Here's the drawing with two shaded views (mm, measured from the low corner). I have some questions. A direction names the side the tool comes from. Coordinates: 2 decimals unless noted, no trailing zeros. Write each loop counter-clockwise with the first axis right and the second up, starting at its lowest first coordinate (ties: lowest second). Pieces come first, ordered by that corner, then holes. Notation, with made-up numbers: (12, 70.5) -> (52, 70.5) arc R14 cw to (52, 92.5) -> close; hole circle Ø4 at (-32, 12.5). An arc over 180 degrees is marked (long way). Put each result on its own line as item: value.
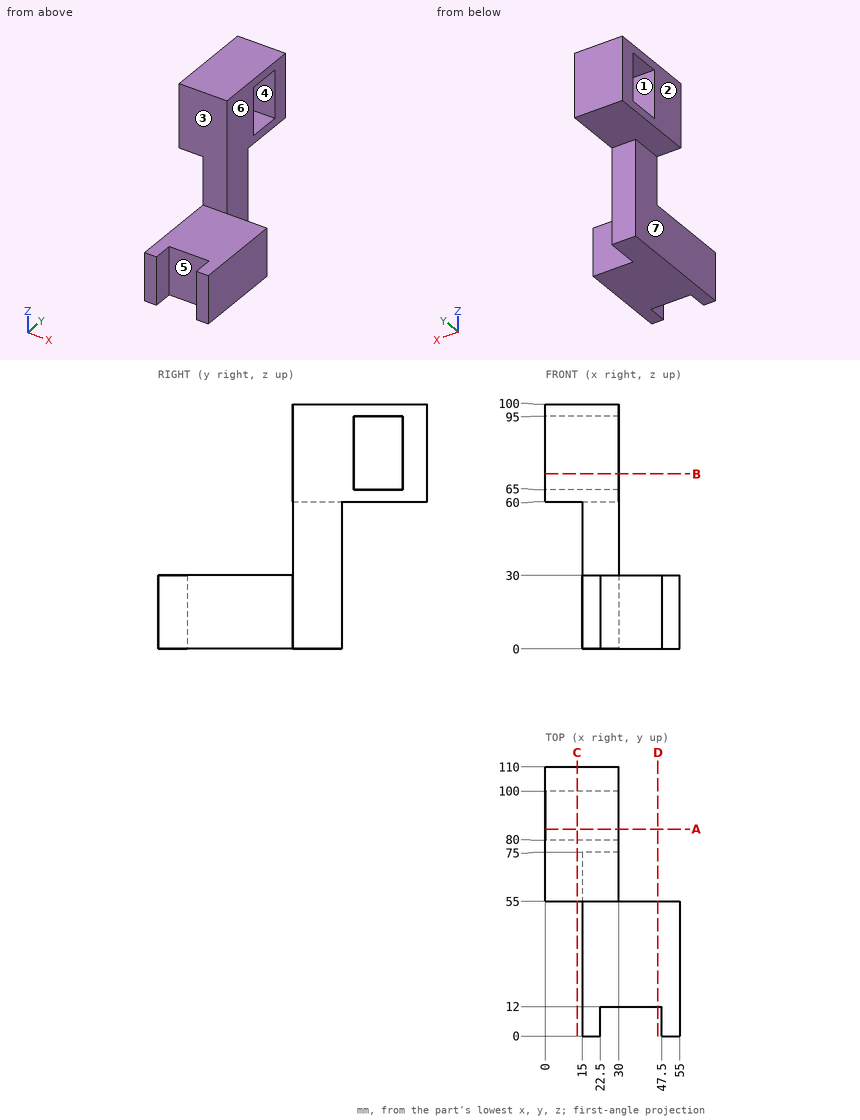
Item 1: For P1, Ø6, axis at y = 58.5, z = 26.5, coming from the +X side; P2, Ø16, axis at x = 9.5, y = 95, coming from the -Z side; P3, Ø15, axis at x = 10.5, z = 51, coming from the -Y side; P4, Ø12, axis at x = 24, z = 32.5, coming from the -Y side, each with a flat end and sliding along its axis, tell me the tip position at first contact or that it passes through.
Output:
P1: stops at x = 30
P2: stops at z = 60
P3: stops at y = 55
P4: stops at y = 0
Item 2: Please list where these lines run through material, in increasing order: line 1 along Y through (x, z) = (15.5, 78); line 2 along Z through (x, y) = (6, 82); line 3 along Z through (x, y) = (23.5, 25.5). Write a range as from..to.
Output:
line 1: y = 55..80, 100..110
line 2: z = 60..65, 95..100
line 3: z = 0..30
Item 3: Imagine slicing it at B-B on z = 71.5. Write out the boundary of the cut face in (x, y), then the cut area to 3 significant figures.
Output:
outline: (0, 55) -> (30, 55) -> (30, 80) -> (0, 80) -> close; (0, 100) -> (30, 100) -> (30, 110) -> (0, 110) -> close
area: 1,050 mm²
Item 4: Imagine slicing it at A-A on y = 84.5. Write out the boundary of the cut face in (x, z), then the cut area to 3 significant figures.
Output:
outline: (0, 60) -> (30, 60) -> (30, 65) -> (0, 65) -> close; (0, 95) -> (30, 95) -> (30, 100) -> (0, 100) -> close
area: 300 mm²
Item 5: If we mould it in two halves opening along Y, with no side actions, what happens to the marked faces 1, 2, 3 and 4? For each: released by +Y, released by -Y, zero draft, split by the parting line, or undercut.
Output:
face 1: undercut
face 2: zero draft
face 3: released by -Y
face 4: undercut
Item 6: Which directions (+Z, -Z, +X, -X, +Y, -Y) give clear straight access to the entire face, cutting with the end or side of a thin tool? Please do the marked faces 5, 6 and 7.
Output:
face 5: +Z, -Z, -Y
face 6: +Z, -Z, +X, +Y
face 7: -Z, -X, +Y, -Y
Item 7: Imagine slicing it at C-C on x = 13. Write out the boundary of the cut face in (y, z).
Output:
outline: (55, 60) -> (110, 60) -> (110, 100) -> (55, 100) -> close; hole (80, 65) -> (100, 65) -> (100, 95) -> (80, 95) -> close
Item 8: Imagine slicing it at D-D on x = 46. Write out the boundary of the cut face in (y, z), then the cut area to 3 significant figures.
Output:
outline: (12, 0) -> (55, 0) -> (55, 30) -> (12, 30) -> close
area: 1,290 mm²
